Can you work these out from the drawing? Everything is in mm from the part's minimum corner. A direction names the side the tool comes from. Give positions to 0.01 mm unless a question says otherwise; leave off trailing zeros. Loops run counter-clockwise (first coordinate to the right, second up) from the corner with the lowest first, then second, coordinate; pieces in that order, holes last.
Q1. We'd pull the mould along Z, two halves only. Please class the marked faces 4, 5, 6 and 7: +Z half, -Z half, draft (parallel to the pull), parting line (faces both ways), or undercut.
Q2. If we section it at D-D (z = 15): Please give me the cut outline in (x, y).
Q3. If we section it at C-C (y = 1.25): Please give me the cut outline in (x, z).
Q4. If we section it at B-B (z = 22): Please give me the cut outline in (x, y).
Q5. I need wall thicknesses on line 1 (Z direction, x = 15, y = 4.25); line 2 (Z direction, x = 38.5, y = 5.5); line 3 (X direction, y = 5.75, z = 15). Which ranges of each line are inside material? Lowest first, please.
Q6. For the marked faces 1, 2 and 3, which set-ups out of +Z, -Z, +X, -X, +Y, -Y let a thin tool reach every point of the face, with its end or its side?
Q7. Will these pins go through, and if not, where does the flat tip stop? P1, Ø12.5, axis at x = 15, z = 15, coming from the +Y side; P2, Ø5, axis at y = 8, z = 8.5, coming from the -X side; P3, Ø5, axis at x = 49, y = 6, coming from the -Z side; P4, Ø3, axis at y = 6, z = 23, coming from the -X side.
Q8. If we section it at A-A (x = 15): Please give me the cut outline in (y, z), plus the area to 3 significant figures.
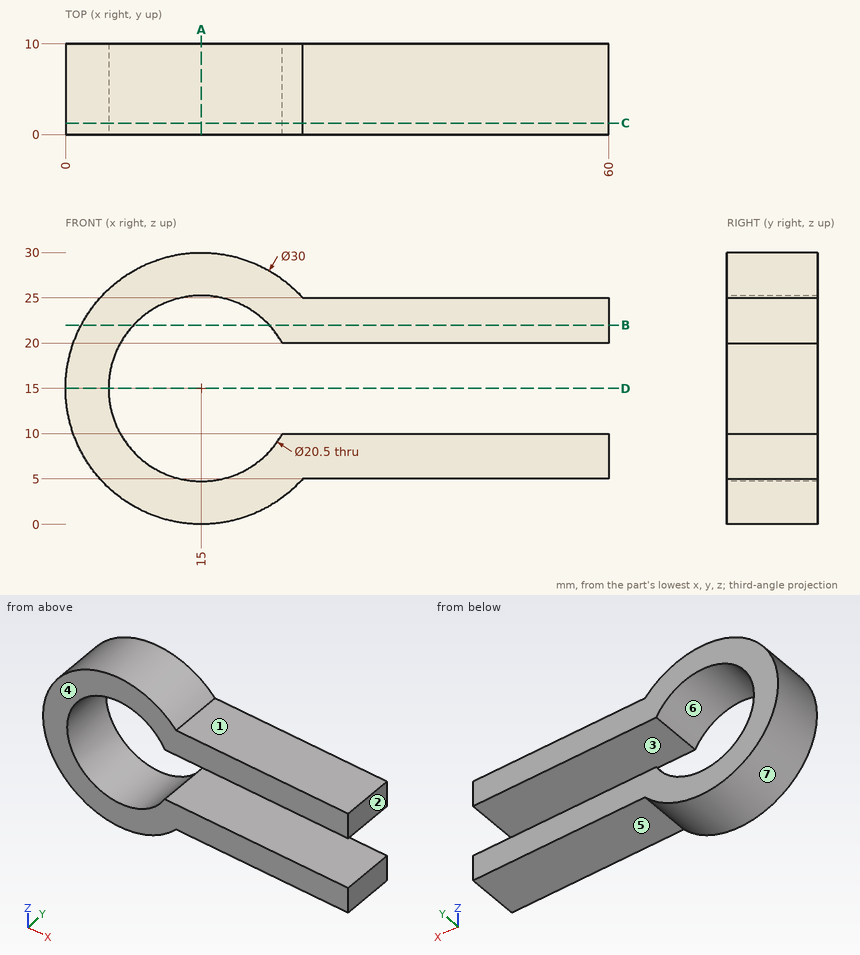
Check sheet entries:
1. face 4: draft
1. face 5: -Z half
1. face 6: undercut
1. face 7: parting line
2. outline: (0, 0) - (4.75, 0) - (4.75, 10) - (0, 10) - close
3. outline: (23.95, 10) arc R10.25 cw (long way) to (23.95, 20) - (60, 20) - (60, 25) - (26.18, 25) arc R15 ccw (long way) to (26.18, 5) - (60, 5) - (60, 10) - close
4. outline: (1.73, 0) - (7.51, 0) - (7.51, 10) - (1.73, 10) - close; (22.49, 0) - (60, 0) - (60, 10) - (22.49, 10) - close
5. line 1: z = 0 to 4.75, 25.25 to 30
5. line 2: z = 5 to 10, 20 to 25
5. line 3: x = 0 to 4.75
6. face 1: +Z, +X, +Y, -Y
6. face 2: +Z, -Z, +X, +Y, -Y
6. face 3: +X, +Y, -Y
7. P1: passes through
7. P2: stops at x = 0.54
7. P3: stops at z = 5
7. P4: stops at x = 1.48
8. outline: (0, 0) - (10, 0) - (10, 4.75) - (0, 4.75) - close; (0, 25.25) - (10, 25.25) - (10, 30) - (0, 30) - close
8. area: 95.0 mm2
